```python
from build123d import *

# Parameters (mm, degrees)
BOSS_EXTRUDE1_DEPTH = 6
SKETCH2_R           = 1.5
CUT_EXTRUDE1_DEPTH  = 3


with BuildPart() as part:
    # Sketch1 → Boss-Extrude1 (new body)
    with BuildSketch(Plane.XY):
        Polygon((-32, 0), (-35, 0), (-35, -20), (0, -20), (0, 0), (-3, 0), (-3, -17), (-32, -17), align=None)
    extrude(amount=BOSS_EXTRUDE1_DEPTH)

    # Sketch2 → Cut-Extrude1 (cut)
    with BuildSketch(Plane.XZ.offset(20)):
        with Locations((-28, 3)):
            Circle(SKETCH2_R)
        with Locations((-7, 3)):
            Circle(SKETCH2_R)
    extrude(amount=-CUT_EXTRUDE1_DEPTH, mode=Mode.SUBTRACT)


solid = part.part
```
Here's how the part is built. I have some questions about the finished solid (model axes, mm). A direction names the side the tool comes from. Give positions to 0.01 mm unless a question says otherwise; leave off trailing zeros. Order: outer loops, then holes, each group sorted by start corner. A loop starts at its lowest first (then second) coordinate and runs counter-clockwise, first axis right, second up. Notation, with made-up numbers: (27, 32.25) -> (78, 32.25) arc R23 ccw to (78, 50.25) -> close; hole circle Ø11 at (56, 87.5). An arc over 180 degrees is marked (long way). Use CSV: the item, a comma, the result in double quotes. Start each with the question number.
Item 1: Suppose I cut it at D-D (z = 1). List the corners of the cut face in (x, y) for me.
Item 2: Thinking about a two-plate mould opening in Z: for faces 3 (the flat face through (-16.3, -17.4, 6)), 4 (the flat face through (-1, 0, 3)), 5 (the flat face through (-16.3, -17.4, 0)), 6 (the cylindrical face through (-8.2, -18.5, 2.1)), which applies, pulls with the +Z half, pulls with the -Z half, needs draft (parallel to the pull), parting line crosses it, or undercut?
Item 3: Suppose I cut it at A-A (y = -16.25). List the corners of the cut face in (x, z) for me.
Item 4: On a 3-axis mill with a long thin cutter (end or side, diameter ignored), from which of +Z, -Z, +X, -X, +Y, -Y can I reach the whole of each face in a straight line? I mean faces 1 (the cylindrical face through (-29.5, -18.52, 3.07)), 2 (the flat face through (-17, -17, 3)). Say none if no direction works.
Item 5: If I drill on probe 1 along Z at (x, y) = (-7, -17.75); probe 2 along X at (y, z) = (-5.5, 5); probe 3 along Y at (x, z) = (-17, 1.95), over which ranges is the centre line in solid material (lowest first)? Write a range as [from, to].
Item 6: I'm going to push flat-ended pins straight in: P1, Ø5, axis at x = -9.5, y = -16, coming from the +Z side; P2, Ø3, axis at x = -8.5, z = 4.5, coming from the +Y side. Where does each tip first touch, or does it pass through?
Item 7: Suppose I cut it at C-C (x = -7). List the corners of the cut face in (y, z) for me.
Item 8: Suppose I cut it at B-B (z = 3). List the corners of the cut face in (x, y) for me, and give its area (3 significant figures).
Answer block:
1,outline,"(-35, -20) -> (0, -20) -> (0, 0) -> (-3, 0) -> (-3, -17) -> (-32, -17) -> (-32, 0) -> (-35, 0) -> close"
2,face 3,"pulls with the +Z half"
2,face 4,"needs draft"
2,face 5,"pulls with the -Z half"
2,face 6,"undercut"
3,outline,"(-35, 0) -> (-32, 0) -> (-32, 6) -> (-35, 6) -> close; (-3, 0) -> (0, 0) -> (0, 6) -> (-3, 6) -> close"
4,face 1,"+Y, -Y"
4,face 2,"+Z, -Z, +Y"
5,probe 1,"z = [0, 1.5], [4.5, 6]"
5,probe 2,"x = [-35, -32], [-3, 0]"
5,probe 3,"y = [-20, -17]"
6,P1,"stops at z = 6"
6,P2,"stops at y = -17"
7,outline,"(-20, 0) -> (-17, 0) -> (-17, 1.5) -> (-20, 1.5) -> close; (-20, 4.5) -> (-17, 4.5) -> (-17, 6) -> (-20, 6) -> close"
8,outline,"(-35, -20) -> (-29.5, -20) -> (-29.5, -17) -> (-32, -17) -> (-32, 0) -> (-35, 0) -> close; (-26.5, -20) -> (-8.5, -20) -> (-8.5, -17) -> (-26.5, -17) -> close; (-5.5, -20) -> (0, -20) -> (0, 0) -> (-3, 0) -> (-3, -17) -> (-5.5, -17) -> close"
8,area,"189 mm^2"
